Autodesk Inventor part; units mm, degrees
ref_plane "YZ Plane" through (0, 0, 0) normal (1, 0, 0) x (0, 1, 0)
ref_plane "XZ Plane" through (0, 0, 0) normal (0, 1, 0) x (-1, 0, 0)
ref_plane "XY Plane" through (0, 0, 0) normal (0, 0, 1) x (1, 0, 0)
sketch "Sketch1" plane through (0, 0, 0) normal (0, 1, 0) x (-1, 0, 0)
  line L0 (3.8, 9.8) -> (-3.8, 9.8)
  line L1 (-3.8, 9.8) -> (-3.8, -9.8)
  line L2 (-3.8, -9.8) -> (3.8, -9.8)
  line L3 (3.8, -9.8) -> (3.8, 9.8)
  circle A0 centre (0, 7.15) radius 1.6
  circle A1 centre (0, -7.15) radius 1.6
  point P0 (0, 0)
  dimension "d0" = 19.6
  dimension "d1" = 7.6
  dimension "d2" = 9.8
  dimension "d3" = 3.8
  dimension "d4" = 3.2
  dimension "d5" = 3.2
  dimension "d6" = 14.3
  dimension "d7" = 7.15
extrude "Extrusion1" add sketch "Sketch1" along normal blind 2.4
fillet "Fillet1" radius 1 4 edges at (3.8, 1.2, 9.8) (-3.8, 1.2, 9.8) (3.8, 1.2, -9.8) (-3.8, 1.2, -9.8)
sketch "Sketch2" plane through (0, 2.4, 0) normal (0, 1, 0) x (1, 0, 0)
  line L0 (-2.35, -2.4313) -> (-2.35, 2.4313)
  line L1 (-2.35, 2.4313) -> (2.35, 4.15)
  line L2 (2.35, 4.15) -> (2.35, -4.15)
  line L3 (2.35, -4.15) -> (-2.35, -2.4313)
  line L4 (1.85, -3.4348) -> (-1.85, -2.0818)
  line L5 (-1.85, -2.0818) -> (-1.85, 2.0818)
  line L6 (-1.85, 2.0818) -> (1.85, 3.4348)
  line L7 (1.85, 3.4348) -> (1.85, -3.4348)
  point P0 (0, 0)
  dimension "d11" = 69.914
  dimension "d13" = 8.3
  dimension "d14" = 4.7
  dimension "d15" = 2.35
  dimension "d17" = 0.5
  dimension "d18" = 0.5
  dimension "d19" = 0.5
  dimension "d20" = 0.5
  dimension "d21" = 4.15
  dimension "d22" = 69.914
  dimension "d23" = 69.914
extrude "Extrusion2" add sketch "Sketch2" along normal blind 4.6
fillet "Fillet2" radius 1 8 edges at (-2.35, 4.7, -2.4313) (-2.35, 4.7, 2.4313) (2.35, 4.7, 4.15) (2.35, 4.7, -4.15) (-1.85, 4.7, -2.0818) (-1.85, 4.7, 2.0818) (1.85, 4.7, -3.4348) (1.85, 4.7, 3.4348)
sketch "Sketch3" plane through (0, 0, 0) normal (0, -1, 0) x (1, 0, 0)
  line L0 (3.4, 4.95) -> (-3.4, 4.95)
  line L1 (-3.4, 4.95) -> (-3.4, -4.95)
  line L2 (-3.4, -4.95) -> (3.4, -4.95)
  line L3 (3.4, -4.95) -> (3.4, 4.95)
  point P0 (0, 0)
  dimension "d27" = 9.9
  dimension "d28" = 6.8
  dimension "d29" = 4.95
  dimension "d30" = 3.4
extrude "Extrusion3" add sketch "Sketch3" along normal blind 3.5
equation "\"d5\" = d4"
equation "\"d22\" = d11"
properties part number "9pin male connector"
Verification items for the finished model (mm, model axes). A direction names the side the tool comes from. Round coordinates to 2 decimals unless told otherwise and drop trailing zeros. Write each loop counter-clockwise with the first axis right and the second up, starting at its lowest first coordinate (ties: lowest second). Pieces come first, ordered by that corner, then holes.
1. Access from +Z, -Z, +X, -X, +Y, -Y to the whole of each face (thin tool, end or side, straight path). Record for faces 1 (the flat face through (0, -2, -4.95)), 2 (the flat face through (2.35, 5, 0)), 3 (the flat face through (0, 2.4, 0)).
2. Scan lines: L1, parallel to Z at x = 0, y = 1.3; L2, parallel to X at y = -0.5, z = 1.25; L3, parallel to Y at x = 0.5, z = -0.5. Record each from-to range of solid material in increasing order.
3. Section check B-B on y = 5. Enter the section's corners in (x, z).
4. Section check A-A on z = 7.15. Enter the section's corners in (x, y).
5. Draft check along Z on faces 4 (the cylindrical face through (1.412, 4.732, 2.832)), 5 (the cylindrical face through (1.934, 4.732, -3.531)), 6 (the flat face through (3.4, -2, 0)). Enter one of: +Z half, -Z half, draft (parallel to the pull), parting line (faces both ways), or undercut.
6. Section check D-D on x = 0. Enter the section's corners in (y, z).
7. Gauge pin test, flat ends, axial feed: P1, Ø3, axis at y = 5.5, z = 1, coming from the -X side; P2, Ø1.1, axis at x = -0.5, z = 1, coming from the +Y side; P3, Ø1.4, axis at y = 5, z = 1, coming from the +X side; P4, Ø2.5, axis at x = 0, z = -7.15, coming from the -Y side. Record the tip position at first contact, or that the pin passes through.
8. Section check C-C on z = 4.75. Enter the section's corners in (x, y), plus the area to 3 significant figures.
Answer:
1. face 1: -Z, +X, -X, -Y
1. face 2: +Z, -Z, +X, +Y
1. face 3: +Y
2. L1: z = -9.8 to -8.75, -5.55 to 5.55, 8.75 to 9.8
2. L2: x = -3.4 to 3.4
2. L3: y = -3.5 to 2.4
3. outline: (-2.35, -1.73) arc R1 ccw to (-1.69, -2.67) - (1.01, -3.66) arc R1 ccw to (2.35, -2.72) - (2.35, 2.72) arc R1 ccw to (1.01, 3.66) - (-1.69, 2.67) arc R1 ccw to (-2.35, 1.73) - close; hole (-1.85, -1.38) arc R1 ccw to (-1.19, -2.32) - (0.51, -2.94) arc R1 ccw to (1.85, -2) - (1.85, 2) arc R1 ccw to (0.51, 2.94) - (-1.19, 2.32) arc R1 ccw to (-1.85, 1.38) - close
4. outline: (-3.8, 0) - (-1.6, 0) - (-1.6, 2.4) - (-3.8, 2.4) - close; (1.6, 0) - (3.8, 0) - (3.8, 2.4) - (1.6, 2.4) - close
5. face 4: undercut
5. face 5: -Z half
5. face 6: draft
6. outline: (-3.5, -4.95) - (0, -4.95) - (0, -5.55) - (2.4, -5.55) - (2.4, -3.29) - (7, -3.29) - (7, -2.76) - (2.4, -2.76) - (2.4, 2.76) - (7, 2.76) - (7, 3.29) - (2.4, 3.29) - (2.4, 5.55) - (0, 5.55) - (0, 4.95) - (-3.5, 4.95) - close; (0, -9.8) - (2.4, -9.8) - (2.4, -8.75) - (0, -8.75) - close; (0, 8.75) - (2.4, 8.75) - (2.4, 9.8) - (0, 9.8) - close
7. P1: stops at x = -2.35
7. P2: stops at y = 2.4
7. P3: stops at x = 2.35
7. P4: passes through
8. outline: (-3.8, 0) - (-3.4, 0) - (-3.4, -3.5) - (3.4, -3.5) - (3.4, 0) - (3.8, 0) - (3.8, 2.4) - (-3.8, 2.4) - close
8. area: 42.0 mm2
